Here's the drawing with two shaded views (mm, measured from the low corner). I have some questions. Coordinates: 2 decimals unless noted, no trailing zeros. Order: outer loops, then holes, each group sorted by start corner. A loop starts at its lowest first (then second) coordinate and runs counter-clockwise, first axis right, second up. Notation, with made-up numbers: (56, -29.75) -> (106, -29.75) arc R17 ccw to (106, 3.25) -> close; hole circle Ø2 at (-39, 70). An arc over 180 degrees is marked (long way). Answer as a JSON object with one key per item and string values. Group by question number.
(1) I need wall thicknesses on line 1 (Y direction, x = 16, z = 13); line 2 (Y direction, x = 13, z = 8.25). Which ranges of each line are inside material? Lowest first, please.
(2) I want a section at A-A, the plane x = 21.5. List the corners of the cut face in (y, z) for me.
(3) For pin 1 (8 mm diameter, centred on x = 10, z = 7.5, fed in from -Y); pin 2 (2 mm diameter, centred on x = 15, z = 21.5, fed in from -Y); pin 3 (6 mm diameter, centred on x = 10, z = 2.5, fed in from -Y), each with a flat end and sliding along its axis, tell me the tip position at first contact or that it passes through.
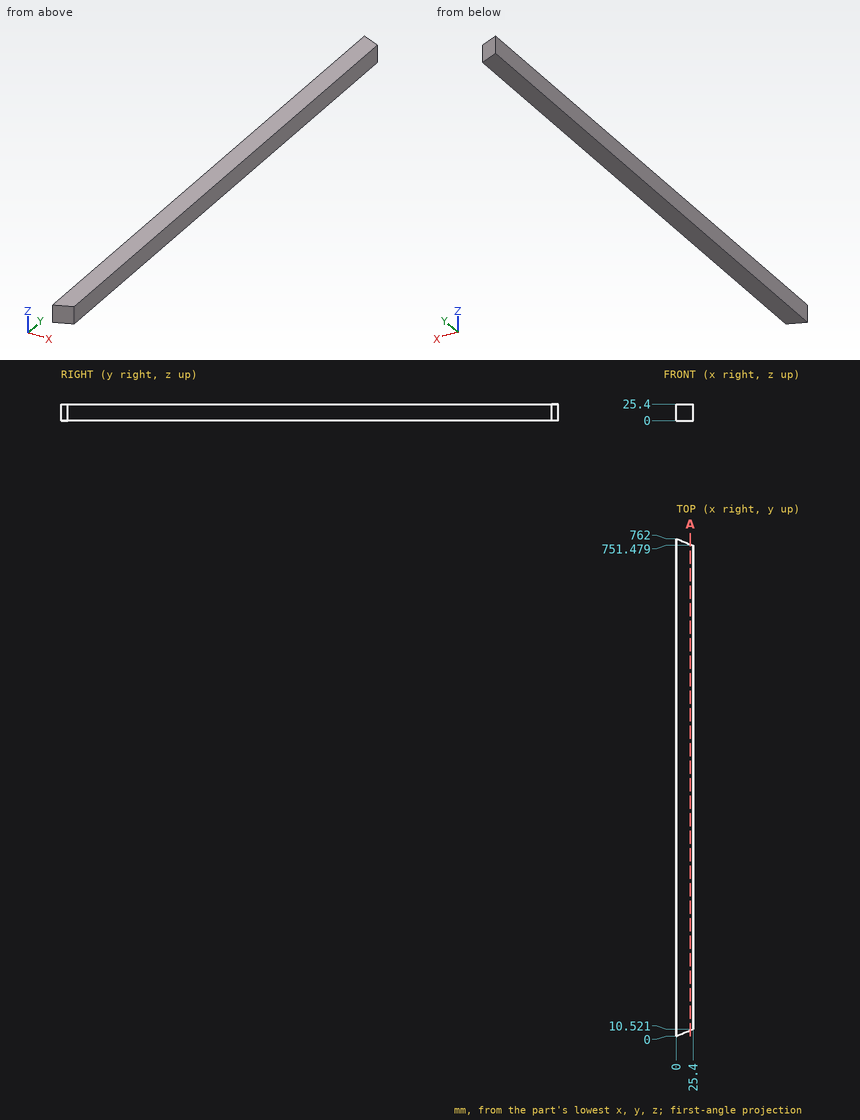
Computed values:
{
 "1": {"line 1": "y = 6.63 to 755.37", "line 2": "y = 5.38 to 756.62"},
 "2": {"outline": "(8.91, 0) -> (753.09, 0) -> (753.09, 25.4) -> (8.91, 25.4) -> close"},
 "3": {"pin 1": "stops at y = 2.49", "pin 2": "stops at y = 5.8", "pin 3": "stops at y = 2.9"}
}
